Input: part model. Units: mm. Frame: model coordinates. Coordinates: 2 decimals unless noted, no trailing zeros. Order: outer loops, then holes, each group sorted by start corner. A loop starts at its lowest first (then second) coordinate and runs counter-clockwise, first axis right, second up. Notation, with made-up numbers: (28, -36.5) - (81, -36.5) arc R25 cw to (81, -5.5) - close; hole circle Ø2 at (-6.5, -18). An arc over 180 degrees is marked (long way). One line per question, with ' | ' between items.
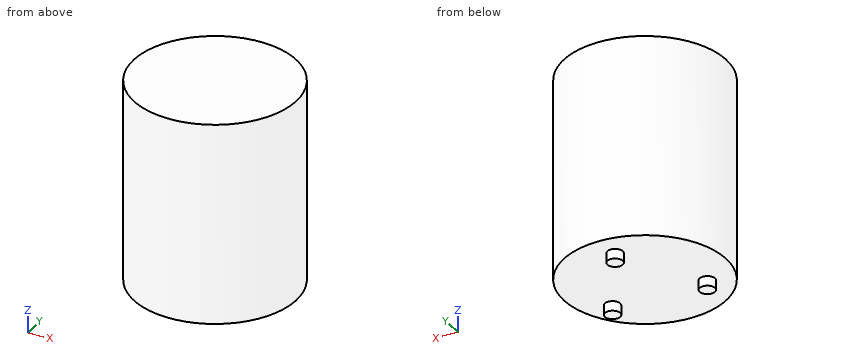
from build123d import *

# Parameters (mm, degrees)
SKETCH1_R           = 21
BOSS_EXTRUDE1_DEPTH = 52
SKETCH2_R           = 2
BOSS_EXTRUDE2_DEPTH = 2.5


with BuildPart() as part:
    # Sketch1 → Boss-Extrude1 (new body)
    with BuildSketch(Plane.XY):
        with Locations(Location((0, 0, 0), (0, 0, 180))):
            Circle(SKETCH1_R)
    extrude(amount=BOSS_EXTRUDE1_DEPTH)

    # Sketch2 → Boss-Extrude2 (add)
    with BuildSketch(Plane.XY):
        with Locations((0, 14.25)):
            Circle(SKETCH2_R)
        with Locations((12.340862004, -7.125)):
            Circle(SKETCH2_R)
        with Locations((-12.340862004, -7.125)):
            Circle(SKETCH2_R)
    extrude(amount=-BOSS_EXTRUDE2_DEPTH)


solid = part.part
Item 1: Ray query, line 1 (Z direction, x = -9, y = -6); line 2 (X direction, y = 11.5, z = 44.5); line 3 (X direction, y = -17, z = 3). Return the intervals inside material, ascending.
Data:
line 1: 0 to 52 | line 2: -17.57 to 17.57 | line 3: -12.33 to 12.33
Item 2: Section C-C on y = 14.25. Return the cut outline in (x, z).
Data:
outline: (-15.43, 0) - (-2, 0) - (-2, -2.5) - (2, -2.5) - (2, 0) - (15.43, 0) - (15.43, 52) - (-15.43, 52) - close
Item 3: Contact query for flat-ended pins moving along their axis: P1, Ø1.5, axis at x = -12.5, z = 5.5, coming from the -Y side; P2, Ø12, axis at x = -11.5, y = 11, coming from the -Z side; P3, Ø5, axis at x = -16.5, z = 44, coming from the +Y side. Output: stop coordinate, or through.
Data:
P1: y = -17.41 | P2: z = 0 | P3: y = 15.65
Item 4: Section A-A on x = 0. Return the cut outline in (y, z).
Data:
outline: (-21, 0) - (12.25, 0) - (12.25, -2.5) - (16.25, -2.5) - (16.25, 0) - (21, 0) - (21, 52) - (-21, 52) - close
Item 5: Section B-B on z = 37. Return the cut outline in (x, y), and give its area (3 significant figures).
Data:
outline: circle Ø42 at (0, 0) | area: 1,390 mm^2
Item 6: Section D-D on x = -4.5. Return the cut outline in (y, z), and give its area (3 significant figures).
Data:
outline: (-20.51, 0) - (20.51, 0) - (20.51, 52) - (-20.51, 52) - close | area: 2,130 mm^2
